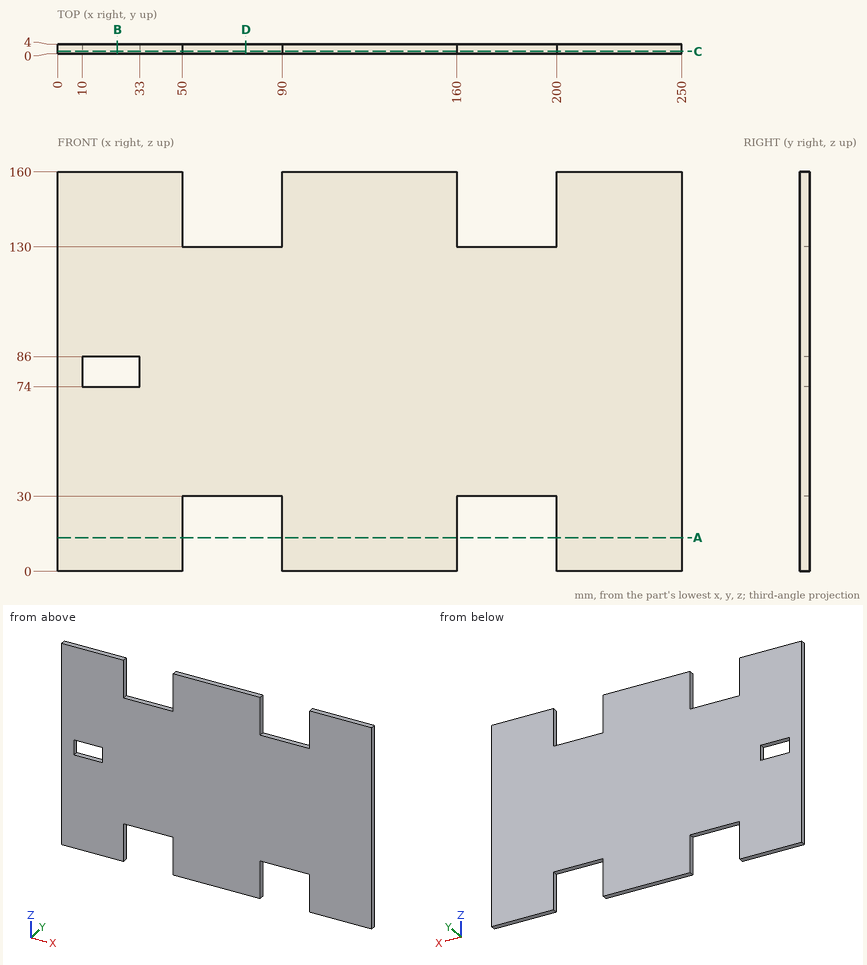
For this review, use the dimensioned drawing (mm, ordinates from the lowest corner) and the shaded views. Round coordinates to 2 decimals unless told otherwise and drop trailing zeros. Loops run counter-clockwise (first coordinate to the right, second up) from the corner with the lowest first, then second, coordinate; pieces in that order, holes last. Notation, with made-up numbers: M -6.5,23 L 15.5,23 A19 ccw 15.5,42 Z; hole C -34,-17.75 d3. An arc over 180 degrees is marked long. Answer as a JSON object with one key per item and string values.
(1) Take a section at A-A on z = 13.5. Give the boundary of the cut face in (x, y), and give its area (3 significant figures).
Resolved:
{"outline": "M 0,0 L 50,0 L 50,4 L 0,4 Z; M 90,0 L 160,0 L 160,4 L 90,4 Z; M 200,0 L 250,0 L 250,4 L 200,4 Z", "area": "680 mm²"}
(2) To check wall thickness, follow line 1 along X through (y, z) = (1.3, 145); line 2 along Z through (x, y) = (11.5, 2.1); line 3 along X through (y, z) = (3.55, 80). State the ranges of each line that lie inside material, in increasing order.
Resolved:
{"line 1": "0 to 50, 90 to 160, 200 to 250", "line 2": "0 to 74, 86 to 160", "line 3": "0 to 10, 33 to 250"}
(3) Take a section at D-D on x = 75.5. Give the boundary of the cut face in (y, z), and give its area (3 significant figures).
Resolved:
{"outline": "M 0,30 L 4,30 L 4,130 L 0,130 Z", "area": "400 mm²"}
(4) Take a section at C-C on y = 1.05. Give the boundary of the cut face in (x, z).
Resolved:
{"outline": "M 0,0 L 50,0 L 50,30 L 90,30 L 90,0 L 160,0 L 160,30 L 200,30 L 200,0 L 250,0 L 250,160 L 200,160 L 200,130 L 160,130 L 160,160 L 90,160 L 90,130 L 50,130 L 50,160 L 0,160 Z; hole M 10,74 L 33,74 L 33,86 L 10,86 Z"}
(5) Take a section at B-B on x = 24. Give the boundary of the cut face in (y, z).
Resolved:
{"outline": "M 0,0 L 4,0 L 4,74 L 0,74 Z; M 0,86 L 4,86 L 4,160 L 0,160 Z"}
(6) Clearance check with flat-ended pins moving along their axes: P1, Ø2, axis at y = 2.5, z = 81.5, coming from the -X side; P2, Ø2, axis at x = 182.5, y = 2, coming from the +Z side; P3, Ø1.2, axis at x = 70, y = 2.5, coming from the -Z side. State where each tip first meets the part, or that it passes through.
Resolved:
{"P1": "x = 0", "P2": "z = 130", "P3": "z = 30"}
